from build123d import *

# Parameters (mm, degrees)
TIGE_START              = -8
ESQUISSE1_R             = 2.5
TIGE_DEPTH              = 8
CHANFREIN_D_ENTR_E_SIZE = 0.5
HEXAGONE_DEPTH          = 1.075


with BuildPart() as part:
    # Esquisse1 → Tige (new body)
    with BuildSketch(Plane(origin=(0, 0, 0), x_dir=(1, 0, 0), z_dir=(0, 1, 0)).offset(TIGE_START)):
        with Locations(Location((0, 0, 0), (0, 0, 270))):
            Circle(ESQUISSE1_R)
    extrude(amount=TIGE_DEPTH)

    # Chanfrein d'entrée
    chanfrein_d_entr_e_edges = [part.edges().sort_by_distance(p)[0] for p in [
        (0, -8, -2.5),
    ]]
    chamfer(chanfrein_d_entr_e_edges, length=CHANFREIN_D_ENTR_E_SIZE)

    # Esquisse2 → Tête (revolve)
    with BuildSketch(Plane.XY, mode=Mode.PRIVATE) as t_te_sk:
        Polygon((0, 0), (4.65, 0), (2.5, -2.15), (0, -2.15), align=None)
    revolve(t_te_sk.sketch.rotate(Axis((0, 0, 0), (0, -1, 0)), 90), axis=Axis((0, 0, 0), (0, -1, 0)))

    # Esquisse3 → Perçage (revolve, cut)
    with BuildSketch(Plane.XY, mode=Mode.PRIVATE) as per_age_sk:
        Polygon((1.5, 0), (1.5, -1.075), (0, -1.941025404), (0, 0), align=None)
    revolve(per_age_sk.sketch.rotate(Axis((0, 0, 0), (0, -1, 0)), 90), axis=Axis((0, 0, 0), (0, -1, 0)), mode=Mode.SUBTRACT)

    # Esquisse5 → Hexagone (cut)
    with BuildSketch(Plane(origin=(0, 0, 0), x_dir=(1, 0, 0), z_dir=(0, 1, 0))):
        Polygon((0.866025404, 1.5), (-0.866025404, 1.5), (-1.732050808, 0), (-0.866025404, -1.5), (0.866025404, -1.5), (1.732050808, 0), align=None)
    extrude(amount=-HEXAGONE_DEPTH, mode=Mode.SUBTRACT)


solid = part.part
The listing builds one solid part. Answer for the finished solid, in the listing's coordinates (mm). A direction names the side the tool comes from. Coordinates: 2 decimals unless noted, no trailing zeros. Order: outer loops, then holes, each group sorted by start corner. A loop starts at its lowest first (then second) coordinate and runs counter-clockwise, first axis right, second up.
Q1. A cutting plane is placed at C-C, the plane y = -1.75. Write down the section's boundary in (x, z).
Q2. A cutting plane is placed at A-A, the plane y = -0.75. Write down the section's boundary in (x, z), and give its area (3 significant figures).
Q3. Consider line 1 (X direction, y = -2.5, z = 0); line 2 (Z direction, x = 2, y = -6.5); line 3 (Z direction, x = 1.5, y = -5.25). Determine where each line is inside the solid, lowest interval first.
Q4. A cutting plane is placed at B-B, the plane y = -6.5. Write down the section's boundary in (x, z), and give its area (3 significant figures).
Q5. Which of the six approach directions +Z, -Z, +X, -X, +Y, -Y give full straight-line access (tool end or side, diameter ignored) to faces 1 (the face through (0, 0, -2)), 2 (the face through (0, -0.5, 1.5))?
Q6. For a pull along Z with two mould halves and no side action, classify faces 3 (the face through (-1.305, -0.53, 0.74)), 4 (the face through (-2.44, -4.86, -0.54)), 5 (the face through (0, -0.5, -1.5)), 6 (the face through (0, -8, 0)) as pulls with the +Z half, pulls with the -Z half, needs draft (parallel to the pull), parting line crosses it, or undercut.
Q7. Given P1, Ø3, axis at x = -3, y = -1, coming from the +Z side; P2, Ø1.5, axis at x = 2, y = -1, coming from the +Z side; P3, Ø2, axis at y = -2.5, z = -1, coming from the +X side, each flat-ended and moving along its own axis, determine where each tip first touches the part or whether it passes through.
Answers follow:
1. outline: circle Ø5.8 at (0, 0); hole circle Ø0.66 at (0, 0)
2. outline: circle Ø7.8 at (0, 0); hole (-1.73, 0) - (-0.87, -1.5) - (0.87, -1.5) - (1.73, 0) - (0.87, 1.5) - (-0.87, 1.5) - close
2. area: 40.0 mm2
3. line 1: x = -2.5 to 2.5
3. line 2: z = -1.5 to 1.5
3. line 3: z = -2 to 2
4. outline: circle Ø5 at (0, 0)
4. area: 19.6 mm2
5. face 1: +Z, -Z, +X, -X, +Y
5. face 2: +Y
6. face 3: undercut
6. face 4: parting line crosses it
6. face 5: undercut
6. face 6: needs draft
7. P1: stops at z = 4.25
7. P2: stops at z = 3.99
7. P3: stops at x = 3.03
